Can you work these out from the model? Positions are in its coordinate system, mm. Face numbers are marked on the shaded views. Coordinates: 2 decimals unless noted, no trailing zeros. Order: outer loops, then holes, each group sorted by start corner. A loop starts at its lowest first (then second) coordinate and runs counter-clockwise, first axis right, second up. Notation, with made-up numbers: (59, -7) -> (84, -7) arc R11 ccw to (84, 2) -> close; hole circle Ø2 at (88.25, 42.5). An arc over 180 degrees is marked (long way). Write item = value, one per line.
```python
from build123d import *

# Parameters (mm, degrees)
SKETCH003_R  = 8.751236
PAD002_DEPTH = 25
SKETCH004_R  = 1.338937
PAD003_DEPTH = 30
SKETCH005_R  = 13.823981
PAD004_DEPTH = 1


with BuildPart() as part:
    # Sketch003 → Pad002 (new body, symmetric)
    with BuildSketch(Plane.XZ):
        Circle(SKETCH003_R)
    extrude(amount=PAD002_DEPTH, both=True)

    # Sketch004 (on Face3 of Pad002) → Pad003 (join)
    with BuildSketch(Plane.XZ.offset(25)):
        Circle(SKETCH004_R)
    extrude(amount=PAD003_DEPTH)

    # Sketch005 (on Face5 of Pad003) → Pad004 (join)
    with BuildSketch(Plane.XZ.offset(55)):
        Circle(SKETCH005_R)
    extrude(amount=PAD004_DEPTH)


with BuildPart() as part_1:
    # Body002 placement: moved
    add(part.part.moved(Location((0, 0, -13))))


solid = part_1.part
```
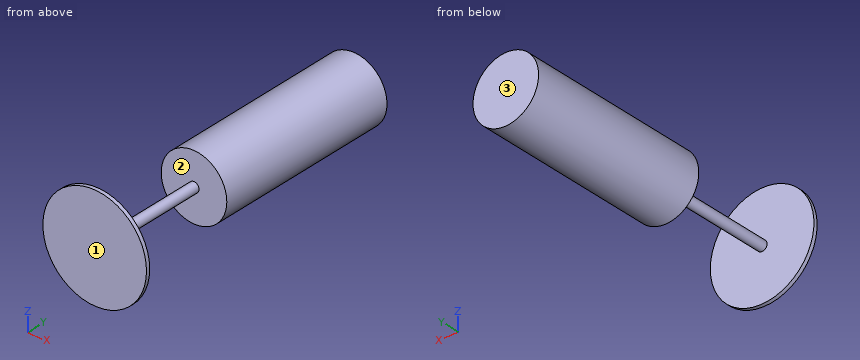
Item 1: I want a section at C-C, the plane x = 0. Please give me the cut outline in (y, z).
A:
outline = (-56, -26.82) -> (-55, -26.82) -> (-55, -14.34) -> (-25, -14.34) -> (-25, -21.75) -> (25, -21.75) -> (25, -4.25) -> (-25, -4.25) -> (-25, -11.66) -> (-55, -11.66) -> (-55, 0.82) -> (-56, 0.82) -> close
Item 2: I want a section at B-B, the plane z = -8.25. Please give me the cut outline in (x, y), plus the area to 3 significant figures.
A:
outline = (-12.98, -56) -> (12.98, -56) -> (12.98, -55) -> (-12.98, -55) -> close; (-7.35, -25) -> (7.35, -25) -> (7.35, 25) -> (-7.35, 25) -> close
area = 761 mm2
Item 3: I'm going to push flat-ended pins straight in: P1, Ø10, axis at y = -1.5, z = -12, coming from the +X side; P2, Ø12, axis at x = -9, y = 6, coming from the +Z side; P3, Ø10, axis at x = 1, y = -2.5, coming from the +Z side. Where does each tip first touch, or does it pass through?
A:
P1 = 8.75
P2 = -4.78
P3 = -4.25
Item 4: If I drill on probe 1 along Y at (x, z) = (-6.75, -18.5); probe 2 along Y at (x, z) = (6.5, -2); probe 3 along X at (y, z) = (12, -19), over which ranges is the centre line in solid material (lowest first)?
A:
probe_1 = -56 to -55, -25 to 25
probe_2 = -56 to -55
probe_3 = -6.37 to 6.37
Item 5: I want a section at D-D, the plane z = -13. Please give me the cut outline in (x, y).
A:
outline = (-13.82, -56) -> (13.82, -56) -> (13.82, -55) -> (1.34, -55) -> (1.34, -25) -> (8.75, -25) -> (8.75, 25) -> (-8.75, 25) -> (-8.75, -25) -> (-1.34, -25) -> (-1.34, -55) -> (-13.82, -55) -> close
Item 6: If we mould it in two halves opening along Y, with no side actions, what happens to the marked faces 1, 2 and 3? For each: pulls with the +Y half, pulls with the -Y half, needs draft (parallel to the pull), parting line crosses it, or undercut.
A:
face_1 = pulls with the -Y half
face_2 = undercut
face_3 = pulls with the +Y half
Item 7: I want a section at A-A, the plane x = -7.5. Please give me the cut outline in (y, z), plus the area to 3 significant figures.
A:
outline = (-56, -24.61) -> (-55, -24.61) -> (-55, -1.39) -> (-56, -1.39) -> close; (-25, -17.51) -> (25, -17.51) -> (25, -8.49) -> (-25, -8.49) -> close
area = 474 mm2
